CAD build for the part. Positions are in the model's coordinates, mm. Coordinates: 2 decimals unless noted, no trailing zeros. Loops run counter-clockwise (first coordinate to the right, second up) from the corner with the lowest first, then second, coordinate; pieces in that order, holes last. Notation, with made-up numbers: (-28.5, 32) - (9.5, 32) arc R9 cw to (9.5, 49) - close; hole circle Ø3 at (71.5, -13.75). An arc over 180 degrees is marked (long way). Put each result on its own line as item: value.
```python
from build123d import *

# Parameters (mm, degrees)
ENL_V_MAT_EXTRU_1_REACH = 3
ESQUISSE3_W             = 0.7
ESQUISSE3_H             = 0.7
BOSS_EXTRU_1_DEPTH      = 24.5
ENL_V_START             = -3.3
ENL_V_MAT_EXTRU_2_DEPTH = 5.9


with BuildPart() as part:
    # Esquisse1 → Révolution1 (revolve)
    with BuildSketch(Plane.XY):
        with BuildLine():
            Line((2.5, 7.6), (2.5, 2.5))
            ThreePointArc((2.5, 2.5), (1.767766953, 0.732233047), (0, 0))
            Line((0, 0), (0, 8.6))
            Line((0, 8.6), (2.95, 8.6))
            Line((2.95, 8.6), (2.95, 7.6))
            Line((2.95, 7.6), (2.5, 7.6))
        make_face()
    revolve(axis=Axis((0, 0, 0), (0, 1, 0)))

    # Esquisse2 → Enlèv. mat.-Extru.1 (cut, up to next)
    with BuildSketch(Plane(origin=(0, 7.6, 0), x_dir=(-1, 0, 0), z_dir=(0, -1, 0)), mode=Mode.PRIVATE) as enl_v_mat_extru_1_sk1:
        Polygon((2.031643218, 2.5), (-2.119175806, 2.5), (-0.304277426, 5.41579693), align=None)
    enl_v_mat_extru_1_tool1 = extrude(enl_v_mat_extru_1_sk1.sketch, amount=-ENL_V_MAT_EXTRU_1_REACH, mode=Mode.PRIVATE) & part.part
    add(enl_v_mat_extru_1_tool1.solids().sort_by_distance((0.130603, 7.6, -3.471932))[0], mode=Mode.SUBTRACT)

    # Esquisse3 → Boss.-Extru.1 (add)
    with BuildSketch(Plane(origin=(0, 8.6, 0), x_dir=(1, 0, 0), z_dir=(0, 1, 0))):
        with Locations((0, 1.905)):
            Rectangle(ESQUISSE3_W, ESQUISSE3_H)
        with Locations((0, -0.635)):
            Rectangle(ESQUISSE3_W, ESQUISSE3_H)
        with Locations((0, -1.905)):
            Rectangle(ESQUISSE3_W, ESQUISSE3_H)
        with Locations((0, 0.635)):
            Rectangle(ESQUISSE3_W, ESQUISSE3_H)
    extrude(amount=BOSS_EXTRU_1_DEPTH)

    # Esquisse4 → Enlèv. mat.-Extru.2 (cut)
    with BuildSketch(Plane.ZY.offset(0.35).offset(ENL_V_START)):
        Polygon((-2.885095567, 30.6), (-1.265657514, 30.6), (-1.265657514, 33.921907916), (0, 33.921907916), (0, 31.83), (1.344412991, 31.83), (1.344412991, 30.6), (2.897512796, 30.6), (2.897512796, 34.676886987), (-2.885095567, 34.676886987), align=None)
    extrude(amount=ENL_V_MAT_EXTRU_2_DEPTH, mode=Mode.SUBTRACT)


solid = part.part
```
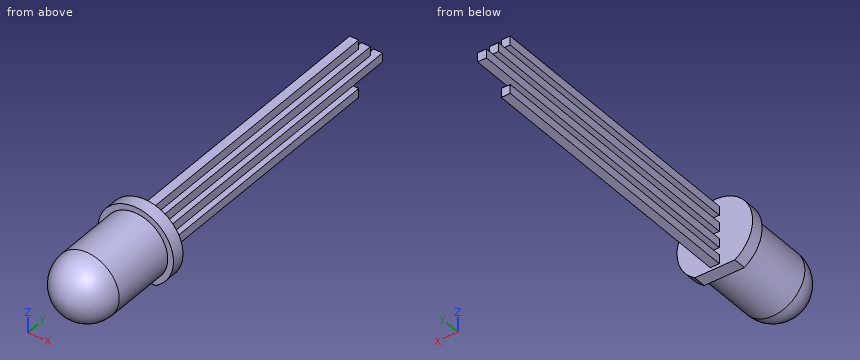
Q1. Slice it at B-B, the plane z = 0. Give the cut face in (x, y), then the cut area to 3 significant figures.
Determined:
outline: (-2.95, 7.6) - (-2.5, 7.6) - (-2.5, 2.5) arc R2.5 ccw to (2.5, 2.5) - (2.5, 7.6) - (2.95, 7.6) - (2.95, 8.6) - (-2.95, 8.6) - close
area: 41.2 mm2
Q2. Slice it at D-D, the plane y = 5. Give the cut face in (x, z).
Determined:
outline: circle Ø5 at (0, 0)
Q3. Pin check, flat tips, straight feed: pin 1 Ø2.5 at (x, z) = (-1.5, 1) entering from -Y; pin 2 Ø0.6 at (y, z) = (16.5, -0.5) entering from +X; pin 3 Ø1 at (y, z) = (16, 0.5) entering from -X. Stop position of each tip, or through.
Determined:
pin 1: y = 0.06
pin 2: x = 0.35
pin 3: x = -0.35
Q4. Slice it at A-A, the plane y = 27.5. Give the cut face in (x, z) (3 decimals).
Determined:
outline: (-0.35, -2.255) - (0.35, -2.255) - (0.35, -1.555) - (-0.35, -1.555) - close; (-0.35, -0.985) - (0.35, -0.985) - (0.35, -0.285) - (-0.35, -0.285) - close; (-0.35, 0.285) - (0.35, 0.285) - (0.35, 0.985) - (-0.35, 0.985) - close; (-0.35, 1.555) - (0.35, 1.555) - (0.35, 2.255) - (-0.35, 2.255) - close
Q5. Wall check: L1, parallel to Z at x = -0.25, y = 15 (3 decimals); L2, parallel to X at y = 30, z = -0.45; L3, parallel to Z at x = 0.05, y = 5.5. Give the ranges that are in metal, low to high. Write a range as from..to.
Determined:
L1: -2.255..-1.555, -0.985..-0.285, 0.285..0.985, 1.555..2.255
L2: -0.35..0.35
L3: -2.5..2.5
Q6. Slice it at C-C, the plane x = 0.95. Give the cut face in (y, z).
Determined:
outline: (2.5, -2.31) - (7.6, -2.31) - (7.6, -2.5) - (8.6, -2.5) - (8.6, 2.79) - (7.6, 2.79) - (7.6, 2.31) - (2.5, 2.31) arc R2.31 ccw to start
